```python
from build123d import *

# Parameters (mm, degrees)
F0_W      = 304.8
F0_H      = 101.6
F1_DEPTH  = 6.35
F3_R      = 14.2875
F4_DEPTH  = 6.35
F5_R      = 3.1115
F9_DEPTH  = 6.35
F6_R      = 3.1115
F10_DEPTH = 6.35
F7_R      = 1.9685
F11_DEPTH = 6.35
F8_R      = 1.9685
F12_DEPTH = 6.35
F15_DEPTH = 6.35
F13_R     = 1.9685
F16_DEPTH = 6.35
F14_R     = 1.9685
F17_DEPTH = 6.35
F18_SIZE  = 50.8
F20_DEPTH = 6.35


with BuildPart() as f1:
    # F0 (on Top) → F1 (new body)
    with BuildSketch(Plane.XY):
        with Locations((79.710026, -8.171286)):
            Rectangle(F0_W, F0_H)
    extrude(amount=F1_DEPTH)

    # F3 (on face) → F4 (cut)
    with BuildSketch(Plane.XY.offset(6.35)):
        with Locations((181.310026, -8.171286)):
            Circle(F3_R)
    extrude(amount=-F4_DEPTH, mode=Mode.SUBTRACT)

    # F5 (on face) → F9 (cut)
    with BuildSketch(Plane.XY.offset(6.35)):
        with Locations((92.410026, 17.863714)):
            Circle(F5_R)
    extrude(amount=-F9_DEPTH, mode=Mode.SUBTRACT)

    # F6 (on face) → F10 (cut)
    with BuildSketch(Plane.XY.offset(6.35)):
        with Locations((92.410026, -34.206286)):
            Circle(F6_R)
    extrude(amount=-F10_DEPTH, mode=Mode.SUBTRACT)

    # F7 (on face) → F11 (cut)
    with BuildSketch(Plane.XY.offset(6.35)):
        with Locations((117.810026, 17.863714)):
            Circle(F7_R)
    extrude(amount=-F11_DEPTH, mode=Mode.SUBTRACT)

    # F8 (on face) → F12 (cut)
    with BuildSketch(Plane.XY.offset(6.35)):
        with Locations((67.010026, 17.863714)):
            Circle(F8_R)
    extrude(amount=-F12_DEPTH, mode=Mode.SUBTRACT)

    # F6 (on face) → F15 (cut)
    with BuildSketch(Plane.XY.offset(6.35)):
        with Locations((92.410026, -34.206286)):
            Circle(F6_R)
    extrude(amount=-F15_DEPTH, mode=Mode.SUBTRACT)

    # F13 (on face) → F16 (cut)
    with BuildSketch(Plane.XY.offset(6.35)):
        with Locations((67.010026, -34.206286)):
            Circle(F13_R)
    extrude(amount=-F16_DEPTH, mode=Mode.SUBTRACT)

    # F14 (on face) → F17 (cut)
    with BuildSketch(Plane.XY.offset(6.35)):
        with Locations((117.810026, -34.206286)):
            Circle(F14_R)
    extrude(amount=-F17_DEPTH, mode=Mode.SUBTRACT)

    # F18
    f18_edges = [f1.edges().sort_by_distance(p)[0] for p in [
        (-72.689974, 42.628714, 3.175),
    ]]
    chamfer(f18_edges, length=F18_SIZE)

    # F19 (on face) → F20 (cut)
    with BuildSketch(Plane(origin=(0, 0, 0), x_dir=(1, 0, 0), z_dir=(0, 0, -1))):
        with BuildLine():
            Line((-33.819589, 5.221926), (-29.329461, 0.731798))
            Line((-29.329461, 0.731798), (-24.839333, 5.221926))
            ThreePointArc((-24.839333, 5.221926), (-29.329461, 7.081798), (-33.819589, 5.221926))
        make_face()
        with BuildLine():
            Line((-24.839333, 5.221926), (-29.329461, 0.731798))
            Line((-29.329461, 0.731798), (-24.839333, -3.75833))
            ThreePointArc((-24.839333, -3.75833), (-23.462826, -1.698242), (-22.979461, 0.731798))
            ThreePointArc((-22.979461, 0.731798), (-23.462826, 3.161838), (-24.839333, 5.221926))
        make_face()
        with BuildLine():
            Line((-29.329461, 0.731798), (-33.819589, -3.75833))
            ThreePointArc((-33.819589, -3.75833), (-29.329461, -5.618202), (-24.839333, -3.75833))
            Line((-24.839333, -3.75833), (-29.329461, 0.731798))
        make_face()
        with BuildLine():
            ThreePointArc((-11.337039, -14.085625), (-13.297019, -11.152307), (-16.757103, -11.840561))
            ThreePointArc((-16.757103, -11.840561), (-15.727059, -17.018942), (-11.337039, -14.085625))
        make_face()
        with BuildLine():
            ThreePointArc((-40.971884, 15.549221), (-47.080201, 16.76424), (-41.90182, 13.304157))
            ThreePointArc((-41.90182, 13.304157), (-41.213566, 14.334201), (-40.971884, 15.549221))
        make_face()
        with BuildLine():
            ThreePointArc((-33.819589, 5.221926), (-35.679461, 0.731798), (-33.819589, -3.75833))
            Line((-33.819589, -3.75833), (-29.329461, 0.731798))
            Line((-29.329461, 0.731798), (-33.819589, 5.221926))
        make_face()
    extrude(amount=-F20_DEPTH, mode=Mode.SUBTRACT)


solid = f1.part
```
Geometry: final body of the model. Coordinates: model frame, mm. Round coordinates to 2 decimals unless told otherwise and drop trailing zeros. Write each loop counter-clockwise with the first axis right and the second up, starting at its lowest first coordinate (ties: lowest second). Pieces come first, ordered by that corner, then holes.
Item 1: Material intervals for L1, parallel to X at y = 4, z = 6.25; L2, parallel to X at y = -15, z = 5.25; L3, parallel to Y at x = 179, z = 2.75, sorted ascending.
Item 2: Section query A-A (x = 180.5). Return loops of the section in (y, z).
Item 3: Section query C-C (y = 31.5). Return loops of the section in (x, z), plus the area to 3 significant figures.
Item 4: Section query D-D (x = -50). Return loops of the section in (y, z).
Item 5: Pin query (flat end, axial travel): P1, Ø8, axis at x = 92.41, y = 17.86, coming from the -Z side; P2, Ø2, axis at y = -4, z = 4.5, coming from the -X side; P3, Ø3, axis at y = 24, z = 1.5, coming from the -X side. Return the tip coordinate at first contact, or that it passes through.
Item 6: Section query B-B (z = 3). Give the number of separate pieces and of enclosed holes in the cut face, plus the area to 3 significant figures.
Item 7: Mould query, pull axis Y, two halves, no side actions, for faces 1 (the face through (232.11, -9, 3)), 2 (the face through (-46.934, 17.584, 3.131)), 3 (the face through (95.378, 18.798, 3.219)). Classes: +Y half, -Y half, draft (parallel to the pull), parting line (faces both ways), or undercut.
Completed:
1. L1: x = -60.52 to -33.56, -25.09 to 173.83, 188.79 to 232.11
1. L2: x = -72.69 to -47.27, -41.02 to 168.76, 193.86 to 232.11
1. L3: y = -58.97 to -22.27, 5.93 to 42.63
2. outline: (-58.97, 0) - (-22.44, 0) - (-22.44, 6.35) - (-58.97, 6.35) - close; (6.09, 0) - (42.63, 0) - (42.63, 6.35) - (6.09, 6.35) - close
3. outline: (-33.02, 0) - (232.11, 0) - (232.11, 6.35) - (-33.02, 6.35) - close
3. area: 1,680 mm2
4. outline: (-58.97, 0) - (14.52, 0) - (14.52, 6.35) - (-58.97, 6.35) - close
5. P1: stops at z = 0
5. P2: stops at x = -69.52
5. P3: stops at x = -42.02
6. separate pieces: 1
6. enclosed holes: 10
6. area: 28,700 mm2
7. face 1: draft
7. face 2: +Y half
7. face 3: undercut
